```python
from build123d import *

# Parameters (mm, degrees)
SCHIZZO1_W                   = 140
SCHIZZO1_H                   = 95.5
ESTRUSIONE_ESTRUSIONE1_DEPTH = 3
SCHIZZO2_R                   = 6
TAGLIO_ESTRUSIONE1_DEPTH     = 3
SCHIZZO3_W                   = 104
SCHIZZO3_H                   = 8
ESTRUSIONE_ESTRUSIONE2_DEPTH = 8
TAGLIO_ESTRUSIONE2_DEPTH     = 104
SCHIZZO5_W                   = 9
SCHIZZO5_H                   = 12
ESTRUSIONE_ESTRUSIONE3_DEPTH = 12
RACCORDO1_R                  = 2
RACCORDO2_R                  = 6.5
SCHIZZO6_R                   = 1.7
TAGLIO_ESTRUSIONE3_DEPTH     = 165.012469038
TAGLIO_ESTRUSIONE4_DEPTH     = 2.5
TAGLIO_ESTRUSIONE5_DEPTH     = 2.5


with BuildPart() as part:
    # Schizzo1 → Estrusione-Estrusione1 (new body)
    with BuildSketch(Plane(origin=(0, 0, 0), x_dir=(1, 0, 0), z_dir=(0, 1, 0))):
        with Locations((70, 47.75)):
            Rectangle(SCHIZZO1_W, SCHIZZO1_H)
    extrude(amount=ESTRUSIONE_ESTRUSIONE1_DEPTH)

    # Schizzo2 → Taglio-Estrusione1 (cut)
    with BuildSketch(Plane(origin=(0, 3, 0), x_dir=(1, 0, 0), z_dir=(0, 1, 0))):
        with Locations(Location((50, 20, 0), (0, 0, 270))):
            Circle(SCHIZZO2_R)
        with Locations(Location((90, 20, 0), (0, 0, 270))):
            Circle(SCHIZZO2_R)
    extrude(amount=-TAGLIO_ESTRUSIONE1_DEPTH, mode=Mode.SUBTRACT)

    # Schizzo3 → Estrusione-Estrusione2 (add)
    with BuildSketch(Plane.XZ):
        with Locations((70, -4)):
            Rectangle(SCHIZZO3_W, SCHIZZO3_H)
    extrude(amount=ESTRUSIONE_ESTRUSIONE2_DEPTH)

    # Schizzo4 → Taglio-Estrusione2 (cut)
    with BuildSketch(Plane(origin=(122, 0, 0), x_dir=(0, 0, -1), z_dir=(1, 0, 0))):
        Polygon((0, 0), (0, -8), (1, -8), (1, -4), (3, -4), (3, 0), align=None)
    extrude(amount=-TAGLIO_ESTRUSIONE2_DEPTH, mode=Mode.SUBTRACT)

    # Schizzo5 → Estrusione-Estrusione3 (add)
    with BuildSketch(Plane.XZ):
        with Locations((11.7, -86.3)):
            Rectangle(SCHIZZO5_W, SCHIZZO5_H)
        with Locations((128.3, -86.3)):
            Rectangle(SCHIZZO5_W, SCHIZZO5_H)
    extrude(amount=ESTRUSIONE_ESTRUSIONE3_DEPTH)

    # Raccordo1
    raccordo1_edges = [part.edges().sort_by_distance(p)[0] for p in [
        (140, 3, -47.75),
        (70, 3, -95.5),
        (0, 3, -47.75),
        (0, 1.5, -95.5),
        (140, 1.5, -95.5),
        (140, 1.5, 0),
        (0, 1.5, 0),
        (70, 3, 0),
    ]]
    fillet(raccordo1_edges, radius=RACCORDO1_R)

    # Raccordo2
    raccordo2_edges = [part.edges().sort_by_distance(p)[0] for p in [
        (11.7, -12, -92.3),
        (128.3, -12, -92.3),
    ]]
    fillet(raccordo2_edges, radius=RACCORDO2_R)

    # Schizzo6 → Taglio-Estrusione3 (cut, through all)
    with BuildSketch(Plane.ZY.offset(-7.2)):
        with Locations((-87.5, -5)):
            Circle(SCHIZZO6_R)
    extrude(amount=-TAGLIO_ESTRUSIONE3_DEPTH, mode=Mode.SUBTRACT)

    # Schizzo7 → Taglio-Estrusione4 (cut)
    with BuildSketch(Plane.ZY.offset(-123.8)):
        Polygon((-90.35, -6.645448267), (-87.5, -8.290896534), (-84.65, -6.645448267), (-84.65, -3.354551733), (-87.5, -1.709103466), (-90.35, -3.354551733), align=None)
    extrude(amount=-TAGLIO_ESTRUSIONE4_DEPTH, mode=Mode.SUBTRACT)

    # Schizzo8 → Taglio-Estrusione5 (cut)
    with BuildSketch(Plane(origin=(16.2, 0, 0), x_dir=(0, 0, -1), z_dir=(1, 0, 0))):
        Polygon((84.65, -6.645448267), (87.5, -8.290896534), (90.35, -6.645448267), (90.35, -3.354551733), (87.5, -1.709103466), (84.65, -3.354551733), align=None)
    extrude(amount=-TAGLIO_ESTRUSIONE5_DEPTH, mode=Mode.SUBTRACT)


solid = part.part
```
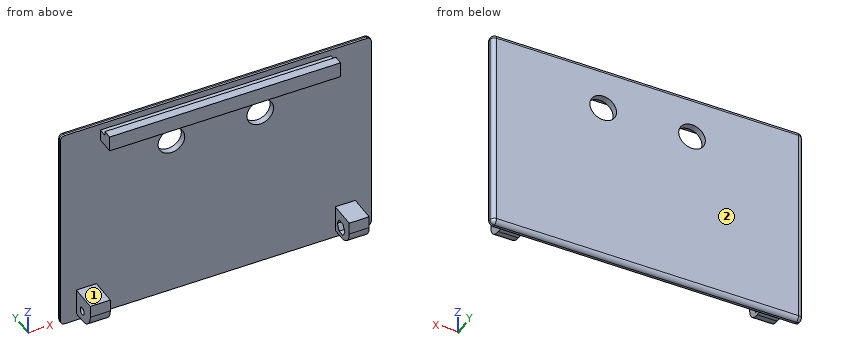
Model file for the job. Use its own axes, mm. Face numbers are marked on the shaded views. A direction names the side the tool comes from. Coordinates: 2 decimals unless noted, no trailing zeros. Write each loop counter-clockwise with the first axis right and the second up, starting at its lowest first coordinate (ties: lowest second). Pieces come first, ordered by that corner, then holes. Notation, with made-up numbers: (1.5, 1.25) - (12.5, 1.25) arc R27 cw to (12.5, 32.25) - close; hole circle Ø8 at (79, -9). An arc over 180 degrees is marked (long way). One line per item, written item: value. Start each with the question number.
1. Probe line 1 (X direction, y = 0.9, z = -20); line 2 (X direction, y = -6, z = -85); line 3 (Z direction, x = 30, y = -6.5). List the from-to ranges inside material, lowest first. Write a range as from..to.
2. Slice it at C-C (z = -43). Write the cut outline in (x, y), plus the area to 3 significant figures.
3. Slice it at A-A (x = 90). Write the cut outline in (y, z).
4. Slice it at B-B (z = -20). Write the cut outline in (x, y).
5. Flat gauge pins, fed straight in: pin 1 (0.8 mm diameter, centred on x = 125.5, y = -5.5, fed in from -Z); pin 2 (1 mm diameter, centred on x = 87, y = -7, fed in from +Z); pin 3 (7.5 mm diameter, centred on y = -4, z = -5, fed in from +X). Where does each tip first touch, or does it go through?
6. Tool access for the marked faces 1 and 2: list every direction of +Z, -Z, +X, -X, +Y, -Y with a clear straight run to the whole face (end or side of a thin tool).
Answers below:
1. line 1: x = 0..44, 56..84, 96..140
1. line 2: x = 7.2..13.7, 126.3..132.8
1. line 3: z = -8..-1
2. outline: (0, 0) - (140, 0) - (140, 1) arc R2 ccw to (138, 3) - (2, 3) arc R2 ccw to (0, 1) - close
2. area: 418 mm^2
3. outline: (-8, -8) - (0, -8) - (0, -14) - (3, -14) - (3, -2) arc R2 ccw to (1, 0) - (0, 0) - (0, -3) - (-4, -3) - (-4, -1) - (-8, -1) - close; (0, -95.5) - (1, -95.5) arc R2 ccw to (3, -93.5) - (3, -26) - (0, -26) - close
4. outline: (0, 0) - (44, 0) - (44, 3) - (2, 3) arc R2 ccw to (0, 1) - close; (56, 0) - (84, 0) - (84, 3) - (56, 3) - close; (96, 0) - (140, 0) - (140, 1) arc R2 ccw to (138, 3) - (96, 3) - close
5. pin 1: stops at z = -92.3
5. pin 2: stops at z = -1
5. pin 3: stops at x = 122
6. face 1: +Z, +X, -X, -Y
6. face 2: +Z, -Z, +X, -X, +Y
